The listing builds one solid part. Answer for the finished solid, in the listing's coordinates (mm). A direction names the side the tool comes from. Round coordinates to 2 decimals unless told otherwise and drop trailing zeros. Loops run counter-clockwise (first coordinate to the right, second up) from the corner with the lowest first, then second, coordinate; pieces in that order, holes last. Notation, with made-up numbers: (28, 9) -> (46, 9) arc R14 cw to (46, 33) -> close; hole circle Ø6 at (7.25, 15). An arc over 180 degrees is marked (long way). Use a Markdown table: item, result. Add a question column.
Q1. Given pin 1 Ø3.5 at (y, z) = (0, 0) entering from +X; pin 2 Ø4 at (y, z) = (0, 0) entering from +X, each flat-ended and moving along its own axis, determine where each tip first touches the part or whether it passes through.
Q2. Which of the six approach directions +Z, -Z, +X, -X, +Y, -Y give full straight-line access (tool end or side, diameter ignored) to faces 1 (the cylindrical face through (3.3, -2.44, -0.54)), 2 (the cylindrical face through (33.507, 1.802, 5.723)), 3 (the cylindrical face through (15.12, -4.88, -1.08)), 4 (the flat face through (14, 0, 6.5)), 5 (the flat face through (13.8, 5.6, -3.3))?
Q3. For a pull along X with two mould halves and no side action, classify faces 6 (the cylindrical face through (32.26, -4.88, -1.08)), 7 (the cylindrical face through (1.479, 4.397, 0.052)), 8 (the flat face through (6.5, -2, -2)), 9 (the flat face through (28, -6, -2)) as released by +X, released by -X, zero draft, split by the parting line, or undercut.
Q4. Section C-C on z = 3.75 is taken. Give the vertices of the cut face in (x, y).
Q5. Section B-B on y = -3 is taken. Give the vertices of the cut face in (x, z), then the cut area to 3 significant figures.
Q6. Consider line 1 (X direction, y = -3.5, z = 4.25); line 2 (X direction, y = 2.5, z = 3); line 3 (Y direction, x = 16.5, z = 0). Determine where each line is inside the solid, lowest interval first.
from build123d import *

# Parameters (mm, degrees)
SKETCH_4_R          = 23.958779716
CUT_EXTRUDE_1_DEPTH = 28
SKETCH_5_R          = 0.4
CUT_EXTRUDE_2_DEPTH = 3


with BuildPart() as part:
    # 草图1 → 旋转1 (revolve)
    with BuildSketch(Plane.XY, mode=Mode.PRIVATE) as revolve_1_sk:
        Polygon((0, 0), (0, 7.5), (28, 7.5), (28, 6), (31.5, 6), (31.5, 5), (33, 5), (33, 6), (34, 6), (34, 0), align=None)
    revolve(revolve_1_sk.sketch.rotate(Axis((34, 0, 0), (-1, 0, 0)), 270), axis=Axis((34, 0, 0), (-1, 0, 0)))

    # 草图2 → 切除-旋转1 (revolve, cut)
    with BuildSketch(Plane.XY, mode=Mode.PRIVATE) as cut_revolve_1_sk:
        Polygon((0, 0), (0, 2.5), (6.5, 2.5), (6.5, 5), (23.5, 5), (23.5, 0), align=None)
    revolve(cut_revolve_1_sk.sketch.rotate(Axis((23.5, 0, 0), (-1, 0, 0)), 270), axis=Axis((23.5, 0, 0), (-1, 0, 0)), mode=Mode.SUBTRACT)

    # 草图3 → 切除-旋转2 (revolve, cut)
    with BuildSketch(Plane.XY, mode=Mode.PRIVATE) as cut_revolve_2_sk:
        Polygon((27.806616994, 0), (29, 2.067), (33.567, 2.067), (34, 2.5), (34, 0), align=None)
    revolve(cut_revolve_2_sk.sketch.rotate(Axis((34, 0, 0), (-1, 0, 0)), 270), axis=Axis((34, 0, 0), (-1, 0, 0)), mode=Mode.SUBTRACT)

    # 草图4 → 切除-拉伸1 (cut)
    with BuildSketch(Plane(origin=(0, 0, 0), x_dir=(0, 0, -1), z_dir=(1, 0, 0))):
        Circle(SKETCH_4_R)
        Polygon((-6.5, -3.75277675), (0, -7.505553499), (6.5, -3.75277675), (6.5, 3.75277675), (0, 7.505553499), (-6.5, 3.75277675), align=None, mode=Mode.SUBTRACT)
    extrude(amount=CUT_EXTRUDE_1_DEPTH, mode=Mode.SUBTRACT)

    # 草图5 → 切除-拉伸2 (cut)
    with BuildSketch(Plane(origin=(0, 0, 0), x_dir=(0, 0, -1), z_dir=(1, 0, 0))):
        with Locations((0, 4)):
            Circle(SKETCH_5_R)
    extrude(amount=CUT_EXTRUDE_2_DEPTH, mode=Mode.SUBTRACT)


solid = part.part
Checked values:
| question | item | result |
|---|---|---|
| 1 | pin 1 | stops at x = 28.82 |
| 1 | pin 2 | stops at x = 28.96 |
| 2 | face 1 | -X |
| 2 | face 2 | +X |
| 2 | face 3 | none |
| 2 | face 4 | +Z, +X, -X, +Y, -Y |
| 2 | face 5 | -Z, +X, -X, +Y |
| 3 | face 6 | undercut |
| 3 | face 7 | zero draft |
| 3 | face 8 | undercut |
| 3 | face 9 | released by +X |
| 4 | outline | (0, -5.34) -> (28, -5.34) -> (28, -4.68) -> (31.5, -4.68) -> (31.5, -3.31) -> (33, -3.31) -> (33, -4.68) -> (34, -4.68) -> (34, 4.68) -> (33, 4.68) -> (33, 3.31) -> (31.5, 3.31) -> (31.5, 4.68) -> (28, 4.68) -> (28, 5.34) -> (0, 5.34) -> close; hole (6.5, -3.31) -> (23.5, -3.31) -> (23.5, 3.31) -> (6.5, 3.31) -> close |
| 5 | outline | (0, -6.5) -> (28, -6.5) -> (28, -5.2) -> (31.5, -5.2) -> (31.5, -4) -> (33, -4) -> (33, -5.2) -> (34, -5.2) -> (34, 5.2) -> (33, 5.2) -> (33, 4) -> (31.5, 4) -> (31.5, 5.2) -> (28, 5.2) -> (28, 6.5) -> (0, 6.5) -> close; hole (6.5, -4) -> (23.5, -4) -> (23.5, 4) -> (6.5, 4) -> close |
| 5 | area | 287 mm2 |
| 6 | line 1 | x = 0 to 31.5, 33 to 34 |
| 6 | line 2 | x = 0 to 6.5, 23.5 to 34 |
| 6 | line 3 | y = -7.5 to -5, 5 to 7.5 |
